Work out the finished part from the listing and answer in its coordinate system (mm). Face numbers are marked on the shaded views. A direction names the side the tool comes from. Coordinates: 2 decimals unless noted, no trailing zeros. Write each loop counter-clockwise with the first axis right and the second up, starting at its lowest first coordinate (ties: lowest second). Pieces come first, ordered by that corner, then holes. Notation, with made-up numbers: (12, 57.5) - (41, 57.5) arc R22 ccw to (41, 68.5) - close; hole circle Ø11 at (-1, -37.75). An arc over 180 degrees is marked (long way). Use a Markdown table: item, result. Add a question column.
(1) The part is cut by section C-C, the plane y = 30. Give the vertices of the cut face in (x, z), then the cut area to 3 significant figures.
(2) The part is cut by section A-A, the plane z = 26.5. Give the vertices of the cut face in (x, y).
(3) A tool of negligible diameter and unlimited length cuts with its end or side. For the marked faces 1, 2, 3, 4 and 5, from which of +Z, -Z, +X, -X, +Y, -Y can it reach the whole face along a straight path? Write none if from no direction.
(4) Find the intervals of material crossed by line 1 (Z direction, x = -22, y = -21.5); line 2 (Y direction, x = 31, z = 28); line 3 (Y direction, x = 60, z = 39), in increasing order. Write a range as from..to.
(5) The part is cut by section D-D, the plane z = 5. Give the vertices of the cut face in (x, y), then the cut area to 3 significant figures.
(6) Given pin 1 Ø10 at (x, y) = (-32.5, 6) entering from +Z; pin 2 Ø5 at (y, z) = (49.5, 11.5) entering from -X; pin 3 Ø1.5 at (y, z) = (-21.5, 17) entering from +X; pin 4 Ø23.5 at (y, z) = (31.5, 25) entering from -X, each flat-ended and moving along its own axis, determine where each tip first touches the part or whether it passes through.
(7) The part is cut by section B-B, the plane x = 52. Give the vertices of the cut face in (y, z), then the cut area to 3 significant figures.
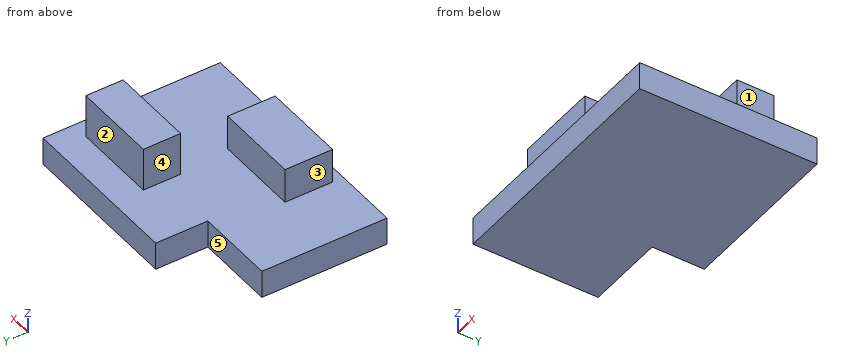
from build123d import *

# Parameters (mm, degrees)
F1_DEPTH = 16
F2_W     = 48.991163
F2_H     = 21.469762
F3_DEPTH = 25
F4_W     = 48.804743
F4_H     = 27.352094
F5_DEPTH = 20


with BuildPart() as f1:
    # F0 (on Top) → F1 (new body)
    with BuildSketch(Plane.XY):
        Polygon((87.884769, 57.809951), (-8.115231, 57.809951), (-8.115231, 27.809951), (-54.115231, 27.809951), (-54.115231, -44.190049), (87.884769, -44.190049), align=None)
    extrude(amount=F1_DEPTH)

    # F2 (on face) → F3 (join)
    with BuildSketch(Plane.XY.offset(16)):
        with Locations((52.972657, 29.482209)):
            Rectangle(F2_W, F2_H)
    extrude(amount=F3_DEPTH)

    # F4 (on face) → F5 (join)
    with BuildSketch(Plane.XY.offset(16)):
        with Locations((7.437617, -24.271876)):
            Rectangle(F4_W, F4_H)
    extrude(amount=F5_DEPTH)


solid = f1.part
Model answer:
| question | item | result |
|---|---|---|
| 1 | outline | (-8.12, 0) - (87.88, 0) - (87.88, 16) - (77.47, 16) - (77.47, 41) - (28.48, 41) - (28.48, 16) - (-8.12, 16) - close |
| 1 | area | 2,760 mm^2 |
| 2 | outline | (-16.96, -37.95) - (31.84, -37.95) - (31.84, -10.6) - (-16.96, -10.6) - close; (28.48, 18.75) - (77.47, 18.75) - (77.47, 40.22) - (28.48, 40.22) - close |
| 3 | face 1 | +Z, +X, +Y, -Y |
| 3 | face 2 | +Z, +X, -X, +Y |
| 3 | face 3 | +Z, -X, +Y, -Y |
| 3 | face 4 | +Z, -X, +Y |
| 3 | face 5 | +Z, -Z, -X, +Y |
| 4 | line 1 | 0..16 |
| 4 | line 2 | -37.95..-10.6, 18.75..40.22 |
| 4 | line 3 | 18.75..40.22 |
| 5 | outline | (-54.12, -44.19) - (87.88, -44.19) - (87.88, 57.81) - (-8.12, 57.81) - (-8.12, 27.81) - (-54.12, 27.81) - close |
| 5 | area | 13,100 mm^2 |
| 6 | pin 1 | z = 16 |
| 6 | pin 2 | x = -8.12 |
| 6 | pin 3 | x = 31.84 |
| 6 | pin 4 | x = -54.12 |
| 7 | outline | (-44.19, 0) - (57.81, 0) - (57.81, 16) - (40.22, 16) - (40.22, 41) - (18.75, 41) - (18.75, 16) - (-44.19, 16) - close |
| 7 | area | 2,170 mm^2 |
